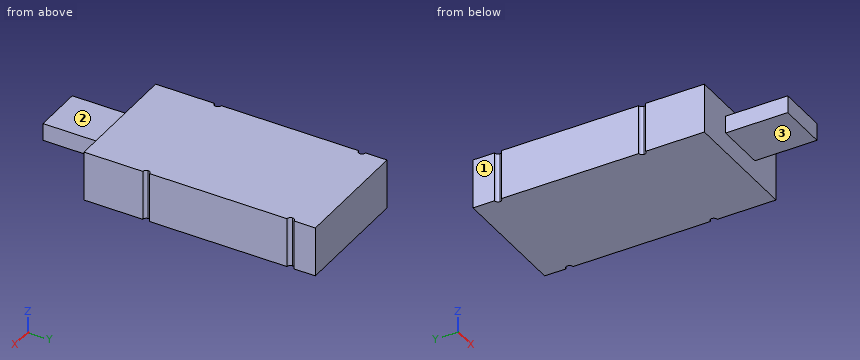
```python
from build123d import *

# Parameters (mm, degrees)
F1_DEPTH = 20
F0_W     = 20
F0_H     = 25
F2_DEPTH = 15
F3_DEPTH = 8


with BuildPart() as f1:
    # F0 (on Top) → F1 (new body)
    with BuildSketch(Plane.XY):
        with BuildLine():
            Line((-14.6488370299, -47.0274474025), (-14.6488370299, 8.2225525975))
            ThreePointArc((-14.6488370299, 8.2225525975), (-15.6211088541, 8.6252807734), (-16.0238370299, 9.5975525975))
            Line((-16.0238370299, 9.5975525975), (-62.2738370299, 9.5975525975))
            ThreePointArc((-62.2738370299, 9.5975525975), (-62.6765652058, 8.6252807734), (-63.6488370299, 8.2225525975))
            Line((-63.6488370299, 8.2225525975), (-63.6488370299, -47.0274474025))
            ThreePointArc((-63.6488370299, -47.0274474025), (-62.6765652058, -47.4301755783), (-62.2738370299, -48.4024474025))
            Line((-62.2738370299, -48.4024474025), (-16.0238370299, -48.4024474025))
            ThreePointArc((-16.0238370299, -48.4024474025), (-15.6211088541, -47.4301755783), (-14.6488370299, -47.0274474025))
        make_face()
        with BuildLine():
            ThreePointArc((-16.0238370299, 9.5975525975), (-15.6211088541, 10.5698244217), (-14.6488370299, 10.9725525975))
            Line((-14.6488370299, 10.9725525975), (-14.6488370299, 19.5975525975))
            Line((-14.6488370299, 19.5975525975), (-63.6488370299, 19.5975525975))
            Line((-63.6488370299, 19.5975525975), (-63.6488370299, 10.9725525975))
            ThreePointArc((-63.6488370299, 10.9725525975), (-62.6765652058, 10.5698244217), (-62.2738370299, 9.5975525975))
            Line((-62.2738370299, 9.5975525975), (-16.0238370299, 9.5975525975))
        make_face()
        with BuildLine():
            ThreePointArc((-14.6488370299, -49.7774474025), (-15.6211088541, -49.3747192266), (-16.0238370299, -48.4024474025))
            Line((-16.0238370299, -48.4024474025), (-62.2738370299, -48.4024474025))
            ThreePointArc((-62.2738370299, -48.4024474025), (-62.6765652058, -49.3747192266), (-63.6488370299, -49.7774474025))
            Line((-63.6488370299, -49.7774474025), (-63.6488370299, -73.4024474025))
            Line((-63.6488370299, -73.4024474025), (-49.1488370299, -73.4024474025))
            Line((-49.1488370299, -73.4024474025), (-29.1488370299, -73.4024474025))
            Line((-29.1488370299, -73.4024474025), (-14.6488370299, -73.4024474025))
            Line((-14.6488370299, -73.4024474025), (-14.6488370299, -49.7774474025))
        make_face()
    extrude(amount=F1_DEPTH)

    # F0 (on Top) → F2 (join)
    with BuildSketch(Plane.XY):
        with Locations((-39.1488370299, -85.9024474025)):
            Rectangle(F0_W, F0_H)
    extrude(amount=F2_DEPTH)

    # F0 (on Top) → F3 (cut)
    with BuildSketch(Plane.XY):
        with Locations((-39.1488370299, -85.9024474025)):
            Rectangle(F0_W, F0_H)
    extrude(amount=F3_DEPTH, mode=Mode.SUBTRACT)


solid = f1.part
```
CAD build for the part. Positions are in the model's coordinates, mm. Face numbers are marked on the shaded views. A direction names the side the tool comes from. Give positions to 0.01 mm unless a question says otherwise; leave off trailing zeros. Write each loop counter-clockwise with the first axis right and the second up, starting at its lowest first coordinate (ties: lowest second). Pieces come first, ordered by that corner, then holes. Notation, with made-up numbers: M -8.5,16 L 26.5,16 A18 cw 26.5,49 Z; hole C -23,78 d5. An arc over 180 degrees is marked long. Return JSON: item names as keys, results as strings. Group by question number.
(1) Drill centre lines: L1, parallel to Y at x = -40.5, z = 18.5; L2, parallel to Z at x = -39, y = -89; L3, parallel to X at y = 9, z = 1.75. Where is each one in solid material? Low to high. Write a range as [from, to].
(2) Band-saw the part on D-D (x = -54). Give the cut face in (y, z).
(3) Flat gauge pins, fed straight in: pin 1 Ø2 at (x, z) = (-35.5, 6.5) entering from -Y; pin 2 Ø2 at (y, z) = (-88.5, 12) entering from +X; pin 3 Ø16 at (x, y) = (-34.5, -91) entering from +Z. Where does each tip first touch, or does it go through?
(4) 3-axis set-ups, long thin cutter, end or side, ignore diameter. For the marked faces 1, 2 and 3: which of +Z, -Z, +X, -X, +Y, -Y reach the whole face in a straight line?
(5) Band-saw the part on B-B (z = 6.5). Give the cut face in (x, y) (3 decimals).
(6) Band-saw the part on C-C (z = 11.5). Give the cut face in (x, y) (3 decimals).
(7) Band-saw the part on A-A (x = -31). Give the cut face in (y, z).
Entries:
{
 "1": {"L1": "y = [-73.4, 19.6]", "L2": "z = [8, 15]", "L3": "x = [-62.41, -15.89]"},
 "2": {"outline": "M -73.4,0 L 19.6,0 L 19.6,20 L -73.4,20 Z"},
 "3": {"pin 1": "stops at y = -73.4", "pin 2": "stops at x = -29.15", "pin 3": "stops at z = 15"},
 "4": {"face 1": "+Z, -Z, -X, +Y, -Y", "face 2": "+Z, +X, -X, -Y", "face 3": "-Z, +X, -X, -Y"},
 "5": {"outline": "M -63.649,-73.402 L -14.649,-73.402 L -14.649,-49.777 A1.375 cw -14.649,-47.027 L -14.649,8.223 A1.375 cw -14.649,10.973 L -14.649,19.598 L -63.649,19.598 L -63.649,10.973 A1.375 cw -63.649,8.223 L -63.649,-47.027 A1.375 cw -63.649,-49.777 Z"},
 "6": {"outline": "M -63.649,-73.402 L -49.149,-73.402 L -49.149,-98.402 L -29.149,-98.402 L -29.149,-73.402 L -14.649,-73.402 L -14.649,-49.777 A1.375 cw -14.649,-47.027 L -14.649,8.223 A1.375 cw -14.649,10.973 L -14.649,19.598 L -63.649,19.598 L -63.649,10.973 A1.375 cw -63.649,8.223 L -63.649,-47.027 A1.375 cw -63.649,-49.777 Z"},
 "7": {"outline": "M -98.4,8 L -73.4,8 L -73.4,0 L 19.6,0 L 19.6,20 L -73.4,20 L -73.4,15 L -98.4,15 Z"}
}
